For this review, take the finished solid that the model builds, in its own axes (mm). A direction names the side the tool comes from. Give positions to 0.01 mm unless a question says otherwise; leave off trailing zeros. Order: outer loops, then holes, each group sorted by start corner. A loop starts at its lowest first (then second) coordinate and runs counter-clockwise, first axis right, second up. Notation, with made-up numbers: (70, 89) - (100, 89) arc R14 ccw to (100, 111) - close; hole circle Ø1 at (-5, 11). An arc over 180 degrees is marked (long way). Answer as a JSON object with one key per item and string values. Group by question number.
from build123d import *

# Parameters (mm, degrees)
F0_R     = 5.1
F0_R_2   = 3.875
F1_DEPTH = 6
F2_START = 4
F0_R_3   = 6.25
F2_DEPTH = 2
F3_SIZE  = 1


with BuildPart() as f1:
    # F0 (on Top) → F1 (new body)
    with BuildSketch(Plane.XY):
        Circle(F0_R)
        Circle(F0_R_2, mode=Mode.SUBTRACT)
    extrude(amount=F1_DEPTH)

    # F0 (on Top) → F2 (join)
    with BuildSketch(Plane.XY.offset(F2_START)):
        Circle(F0_R_3)
        Circle(F0_R, mode=Mode.SUBTRACT)
    extrude(amount=F2_DEPTH)

    # F3
    f3_edges = [f1.edges().sort_by_distance(p)[0] for p in [
        (-6.25, 0, 6),
    ]]
    chamfer(f3_edges, length=F3_SIZE)


solid = f1.part
1) Consider section D-D (z = 2.1). Give the boundary of the cut face in (x, y) (3 decimals).
2) For faces 1 (the face through (2.4, -4.5, 2)), 2 (the face through (-2, -3.5, 6)), list the 3-axis set-ups (+Z, -Z, +X, -X, +Y, -Y) from which the entire face can be reached by the end or side of a thin tool; tool diameter is ignored.
3) Consider section C-C (z = 4.45). Give the boundary of the cut face in (x, y) (3 decimals), plus the area to 3 significant figures.
4) For line 1 (Y direction, x = 0, z = 1.9) (3 decimals); line 2 (Y direction, x = 0, z = 4.55) (3 decimals); line 3 (X direction, y = 2.5, z = 3.65), list the stretches that pass through material, from the lowest coordinate up.
5) Consider section A-A (x = 0). Give the boundary of the cut face in (y, z) (3 decimals).
6) Mouldability with a two-part tool opening along Y and no side actions: class faces 3 (the face through (-2, -5, 4)), 4 (the face through (-0.504, 3.842, 2.958)), 5 (the face through (5.96, 1.88, 4.49)) as released by +Y, released by -Y, zero draft, split by the parting line, or undercut.
7) For pin 1 (1 mm diameter, centred on x = 0.5, z = 1.5, fed in from -Y); pin 2 (3 mm diameter, centred on y = -4, z = 5.5, fed in from -X); pin 3 (2 mm diameter, centred on y = -1, z = 3.5, fed in from +X), all flat-tipped, find the tip position at first contact; note any pin that passes through.
Result set:
{
 "1": {"outline": "circle Ø10.2 at (0, 0); hole circle Ø7.75 at (0, 0)"},
 "2": {"face 1": "-Z", "face 2": "+Z, +X, -X, +Y, -Y"},
 "3": {"outline": "circle Ø12.5 at (0, 0); hole circle Ø7.75 at (0, 0)", "area": "75.5 mm2"},
 "4": {"line 1": "y = -5.1 to -3.875, 3.875 to 5.1", "line 2": "y = -6.25 to -3.875, 3.875 to 6.25", "line 3": "x = -4.45 to -2.96, 2.96 to 4.45"},
 "5": {"outline": "(-6.25, 4) - (-5.1, 4) - (-5.1, 0) - (-3.875, 0) - (-3.875, 6) - (-5.25, 6) - (-6.25, 5) - close; (3.875, 0) - (5.1, 0) - (5.1, 4) - (6.25, 4) - (6.25, 5) - (5.25, 6) - (3.875, 6) - close"},
 "6": {"face 3": "zero draft", "face 4": "undercut", "face 5": "split by the parting line"},
 "7": {"pin 1": "stops at y = -5.1", "pin 2": "stops at x = -5.69", "pin 3": "stops at x = 6.25"}
}
